The model under review builds one solid part; all positions refer to its coordinate system, in mm. Round coordinates to 2 decimals unless told otherwise and drop trailing zeros. Write each loop counter-clockwise with the first axis right and the second up, starting at its lowest first coordinate (ties: lowest second). Pieces come first, ordered by that corner, then holes. Notation, with made-up numbers: M 43.25,-3 L 83.25,-3 A28 ccw 83.25,23 Z; hole C 32.25,40.5 d10. An arc over 180 degrees is marked long. Write item = value, one per line. Start each with the question number.
Item 1: Take a section at C-C, the plane z = 0.4. Give the number of separate pieces and of enclosed holes in the cut face, plus the area to 3 significant figures.
Item 2: For pin 1 Ø1.5 at (y, z) = (10.5, 0.5) entering from +X; pin 2 Ø1.5 at (y, z) = (5.5, 0.5) entering from +X; pin 3 Ø1.5 at (x, z) = (5, 2.5) entering from +Y, all flat-tipped, find the tip position at first contact; note any pin that passes through.
Item 3: Take a section at B-B, the plane y = 0.5. Give the boundary of the cut face in (x, z), plus the area to 3 significant figures.
Item 4: Take a section at A-A, the plane x = 0. Give the boundary of the cut face in (y, z).
Item 5: The part is to be moulded in two halves that separate along Y. For faces 1 (the cylindrical face through (0, 15, 2)), 2 (the cylindrical face through (5.05, -14.29, 1.48)), 3 (the flat face through (-8, 8, 3)), say which applies: +Y half, -Y half, draft (parallel to the pull), parting line (faces both ways), or undercut.
Item 6: To check wall thickness, follow line 1 along Y through (x, z) = (0, 1.05); line 2 along X through (y, z) = (6, 2.4); line 3 along X through (y, z) = (-4, 1.75). State the ranges of each line that lie inside material, in increasing order.
Autodesk Inventor part; units mm, degrees
ref_plane "YZ Plane" through (0, 0, 0) normal (1, 0, 0) x (0, 1, 0)
ref_plane "XZ Plane" through (0, 0, 0) normal (0, 1, 0) x (-1, 0, 0)
ref_plane "XY Plane" through (0, 0, 0) normal (0, 0, 1) x (1, 0, 0)
sketch "スケッチ1" plane through (0, 0, 0) normal (0, 0, 1) x (1, 0, 0)
  circle A0 centre (0, 0) radius 15.5 construction
  circle A1 centre (-16.7262, 17.2115) radius 1.6
  circle A2 centre (0.3431, 23.9975) radius 1.6
  circle A3 centre (17.2115, 16.7262) radius 1.6
  circle A4 centre (23.9975, -0.3431) radius 1.6
  circle A5 centre (16.7262, -17.2115) radius 1.6
  circle A6 centre (-0.3431, -23.9975) radius 1.6
  circle A7 centre (-17.2115, -16.7262) radius 1.6
  circle A8 centre (-23.9975, 0.3431) radius 1.6
  circle A9 centre (0, 0) radius 27.5
  circle A10 centre (0, 0) radius 5.1
  circle A11 centre (4.9497, -4.9497) radius 1.1
  circle A12 centre (7, 0) radius 1.1
  circle A13 centre (4.9497, 4.9497) radius 1.1
  circle A14 centre (0, 7) radius 1.1
  circle A15 centre (-4.9497, 4.9497) radius 1.1
  circle A16 centre (-7, 0) radius 1.1
  circle A17 centre (-4.9497, -4.9497) radius 1.1
  circle A18 centre (0, -7) radius 1.1
  circle A19 centre (0, 0) radius 20.5
  circle A20 centre (0, 0) radius 10.75
  line L0 (0, 0) -> (13.125, 0) construction
  line L1 (9.2808, -9.2808) -> (0, 0) construction
  line L2 (0, 0) -> (12.7033, -5.2619) construction
  circle A21 centre (12.7033, -5.2619) radius 1.6
  circle A22 centre (0, 0) radius 16.75
  line L3 (0, 0) -> (0, -8.1)
  line L4 (0, -10.75) -> (0, -16.75)
  circle A23 centre (0, 0) radius 13.75 construction
  circle A24 centre (12.7033, 5.2619) radius 1.6
  circle A25 centre (0, 0) radius 13.75 construction
  circle A26 centre (5.2619, 12.7033) radius 1.6
  circle A27 centre (0, 0) radius 13.75 construction
  circle A28 centre (-5.2619, 12.7033) radius 1.6
  circle A29 centre (0, 0) radius 13.75 construction
  circle A30 centre (-12.7033, 5.2619) radius 1.6
  circle A31 centre (0, 0) radius 13.75 construction
  circle A32 centre (-12.7033, -5.2619) radius 1.6
  circle A33 centre (0, 0) radius 13.75 construction
  circle A34 centre (-5.2619, -12.7033) radius 1.6
  circle A35 centre (0, 0) radius 13.75 construction
  circle A36 centre (5.2619, -12.7033) radius 1.6
  circle A37 centre (0, 0) radius 13.75 construction
  dimension "d14" = 21.5
  dimension "d15" = 33.5
  dimension "d0" = 13.75
  dimension "d1" = 22.5
  dimension "d2" = 3.2
  dimension "d18" = 27.5
  dimension "d21" = 360
extrude "押し出し3" add sketch "スケッチ1" along normal blind 3 contours A22
sketch "スケッチ2" plane through (0, 0, 3) normal (0, 0, 1) x (1, 0, 0)
  circle A0 centre (0, 0) radius 16.75
  circle A1 centre (5.2619, -12.7033) radius 1.6
  circle A2 centre (0, 0) radius 13.75 construction
  line L0 (0, 0) -> (5.2619, -12.7033)
  line L1 (0, 0) -> (-5.2619, -12.7033)
  line L2 (0, -13.75) -> (0, 0) construction
  circle A3 centre (0, -13.75) radius 1.25
  circle A4 centre (9.7227, -9.7227) radius 1.25
  circle A5 centre (13.75, 0) radius 1.25
  circle A6 centre (9.7227, 9.7227) radius 1.25
  circle A7 centre (0, 13.75) radius 1.25
  circle A8 centre (-9.7227, 9.7227) radius 1.25
  circle A9 centre (-13.75, 0) radius 1.25
  circle A10 centre (-9.7227, -9.7227) radius 1.25
  dimension "d25" = 2.5
  dimension "d28" = 360
extrude "押し出し4" cut sketch "スケッチ2" against normal through all contours A3 | A4 | A5 | A6 | A7 | A8 | A9 | A10
properties part number "出力部品B_ダブルスラスト用(t2_アルミ)" material "アルミニウム 6061"
Response values:
q1.separate_pieces = 1
q1.enclosed_holes = 17
q1.area = 415 mm2
q2.pin_1 = 13.62
q2.pin_2 = 16.06
q2.pin_3 = 16.2
q3.outline = M -16.74,0 L -14.9,0 L -14.9,3 L -16.74,3 Z; M -12.6,0 L -10.74,0 L -10.74,3 L -12.6,3 Z; M 10.74,0 L 12.6,0 L 12.6,3 L 10.74,3 Z; M 14.9,0 L 16.74,0 L 16.74,3 L 14.9,3 Z
q3.area = 22.3 mm2
q4.outline = M -16.75,0 L -15,0 L -15,3 L -16.75,3 Z; M -12.5,0 L -10.75,0 L -10.75,3 L -12.5,3 Z; M 10.75,0 L 12.5,0 L 12.5,3 L 10.75,3 Z; M 15,0 L 16.75,0 L 16.75,3 L 15,3 Z
q5.face_1 = undercut
q5.face_2 = undercut
q5.face_3 = draft
q6.line_1 = -16.75 to -15, -12.5 to -10.75, 10.75 to 12.5, 15 to 16.75
q6.line_2 = -15.64 to -14.12, -11.28 to -8.92, 8.92 to 11.28, 14.12 to 15.64
q6.line_3 = -16.27 to -13.69, -11.72 to -9.98, 9.98 to 11.72, 13.69 to 16.27
